Could you check a few things on this model? Use its own coordinates, in mm. A direction names the side the tool comes from. Round coordinates to 2 decimals unless told otherwise and drop trailing zeros. Write each loop counter-clockwise with the first axis right and the second up, starting at its lowest first coordinate (ties: lowest second). Pieces come first, ordered by that corner, then holes. Notation, with made-up numbers: (78.5, -9.5) - (109.5, -9.5) arc R18 cw to (109.5, 9.5) - close; hole circle Ø1 at (12.5, 87). An arc over 180 degrees is marked (long way). Write each question's results on one line, items separated by ' | '. Start each with the question number.
(1) Imagine slicing it at C-C on y = 234. Write out the boundary of the cut face in (x, z).
(2) Imagine slicing it at B-B on x = 44. Write out the boundary of the cut face in (y, z).
(3) On a 3-axis mill with a long thin cutter (end or side, diameter ignored), from which of +Z, -Z, +X, -X, +Y, -Y can I reach the whole of each face in a straight line? I mean faces 1 (the flat face through (-34, 351, 90)), 2 (the flat face through (-1, 505, 0)), 3 (the flat face through (0, 352, 140)), 4 (the flat face through (-3, 0, 113)). Say none if no direction works.
(4) Imagine slicing it at D-D on z = 199. Write out the boundary of the cut face in (x, y), then the cut area to 3 significant figures.
(5) Imagine slicing it at A-A on z = 82. Write out the boundary of the cut face in (x, y), then the cut area to 3 significant figures.
(6) Please list where these lines run through material, in increasing order: line 1 (X direction, y = 349.5, z = 15); line 2 (Y direction, x = 80, z = 196.5); line 3 (Z direction, x = -134, y = 245.5). Write a range as [from, to].
(7) For P1, Ø4, axis at x = 57.5, z = -10.5, coming from the +Y side; P2, Ø1.5, axis at x = -30.5, y = 119, coming from the +Z side; P3, Ø12, axis at x = -159, z = 174, coming from the +Y side, each with a flat end and sliding along its axis, tell me the tip position at first contact or that it passes through.
```python
from build123d import *

# Parameters (mm, degrees)
SKETCH1_W           = 485
SKETCH1_H           = 500
BOSS_EXTRUDE1_DEPTH = 50
SKETCH2_W           = 485
SKETCH2_H           = 280
BOSS_EXTRUDE2_DEPTH = 17.5


with BuildPart() as part:
    # Sketch1 → Boss-Extrude1 (new body)
    with BuildSketch(Plane.XY):
        with Locations((0, 250)):
            Rectangle(SKETCH1_W, SKETCH1_H)
    extrude(amount=-BOSS_EXTRUDE1_DEPTH)

    # Sketch2 → Boss-Extrude2 (add)
    with BuildSketch(Plane(origin=(0, 0, 0), x_dir=(1, 0, 0), z_dir=(0, 1, 0))):
        with Locations((0, -90)):
            Rectangle(SKETCH2_W, SKETCH2_H)
    extrude(amount=-BOSS_EXTRUDE2_DEPTH)

    # Sketch6 → Revolve1 (revolve)
    with BuildSketch(Plane(origin=(0, 352.6, 0), x_dir=(1, 0, 0), z_dir=(0, 1, 0)), mode=Mode.PRIVATE) as revolve1_sk:
        with BuildLine():
            Line((0, 0), (160, 0))
            Line((160, 0), (160, -40))
            Line((160, -40), (80, -40))
            Line((80, -40), (80, -90))
            Line((80, -90), (30, -90))
            add(Edge.make_bspline(
                [(30, -90), (19.305392217, -92.013307308), (16, -123.873269223), (16, -140)],
                knots=[0, 0, 0, 0, 1, 1, 1, 1], degree=3))
            Line((16, -140), (15.691041026, -140))
            Line((15.691041026, -140), (0, -140))
            Line((0, -140), (0, 0))
        make_face()
    revolve(revolve1_sk.sketch.rotate(Axis((0, 352.6, 0), (0, 0, 1)), 180), axis=Axis((0, 352.6, 0), (0, 0, 1)))


solid = part.part
```
Response:
1) outline: (-242.5, -50) - (242.5, -50) - (242.5, 0) - (107.4, 0) - (107.4, 40) - (-107.4, 40) - (-107.4, 0) - (-242.5, 0) - close
2) outline: (-17.5, -50) - (500, -50) - (500, 0) - (506.43, 0) - (506.43, 40) - (419.41, 40) - (419.41, 90) - (285.79, 90) - (285.79, 40) - (198.77, 40) - (198.77, 0) - (0, 0) - (0, 230) - (-17.5, 230) - close
3) face 1: +Z | face 2: -Z, +X, -X, +Y | face 3: +Z, +X, -X, +Y | face 4: +Z, +X, -X
4) outline: (-242.5, -17.5) - (242.5, -17.5) - (242.5, 0) - (-242.5, 0) - close | area: 8,490 mm²
5) outline: (-242.5, -17.5) - (242.5, -17.5) - (242.5, 0) - (-242.5, 0) - close; circle Ø160 at (0, 352.6) | area: 28,600 mm²
6) line 1: [-159.97, 159.97] | line 2: [-17.5, 0] | line 3: [-50, 0]
7) P1: y = 500 | P2: z = 0 | P3: y = 0
